Answer from the drawing. Dimensions are ordinates in mm from the lowest x, y and z of the part. A direction names the side the tool comes from. Coordinates: 2 decimals unless noted, no trailing zeros. Order: outer loops, then holes, each group sorted by start corner. A loop starts at its lowest first (then second) coordinate and runs counter-clockwise, first axis right, second up. Notation, with made-up numbers: (34.25, 41.25) - (45.25, 41.25) arc R27 ccw to (45.25, 72.25) - close; hole circle Ø9 at (53, 34.5). An arc over 180 degrees is marked (long way). Use a Markdown table: item, result. Add a question column.
Item 1: The part is cut by section A-A, the plane y = 11.5. Give the vertices of the cut face in (x, z) (1 decimal).
Item 2: Flat-ended cylindrical pins translate along their axes: P1, Ø5, axis at x = 44, z = 42, coming from the -Y side; P2, Ø8, axis at y = 14.5, z = 35, coming from the +X side; P3, Ø2, axis at x = 26.5, z = 53, coming from the -Y side (1 decimal). Find the tip coordinate at first contact, or state that the pin passes through.
Item 3: For the marked faces 4 and 5, determine the directions among +Z, -Z, +X, -X, +Y, -Y from which every point of the face is accessible in a straight line to the end or side of a thin tool.
Item 4: The part is cut by section D-D, the plane y = 15.75. Give the vertices of the cut face in (x, z) (1 decimal).
Item 5: Find the intervals of material crossed by line 1 along Z through (x, y) = (55.5, 25.25); line 2 along Z through (x, y) = (9, 9) (1 decimal); line 3 along X through (y, z) = (23.75, 32.5) (1 decimal), in increasing order.
Item 6: The mould has two halves that part along X. Classify the marked faces 1, 2 and 3: released by +X, released by -X, zero draft, split by the parting line, or undercut.
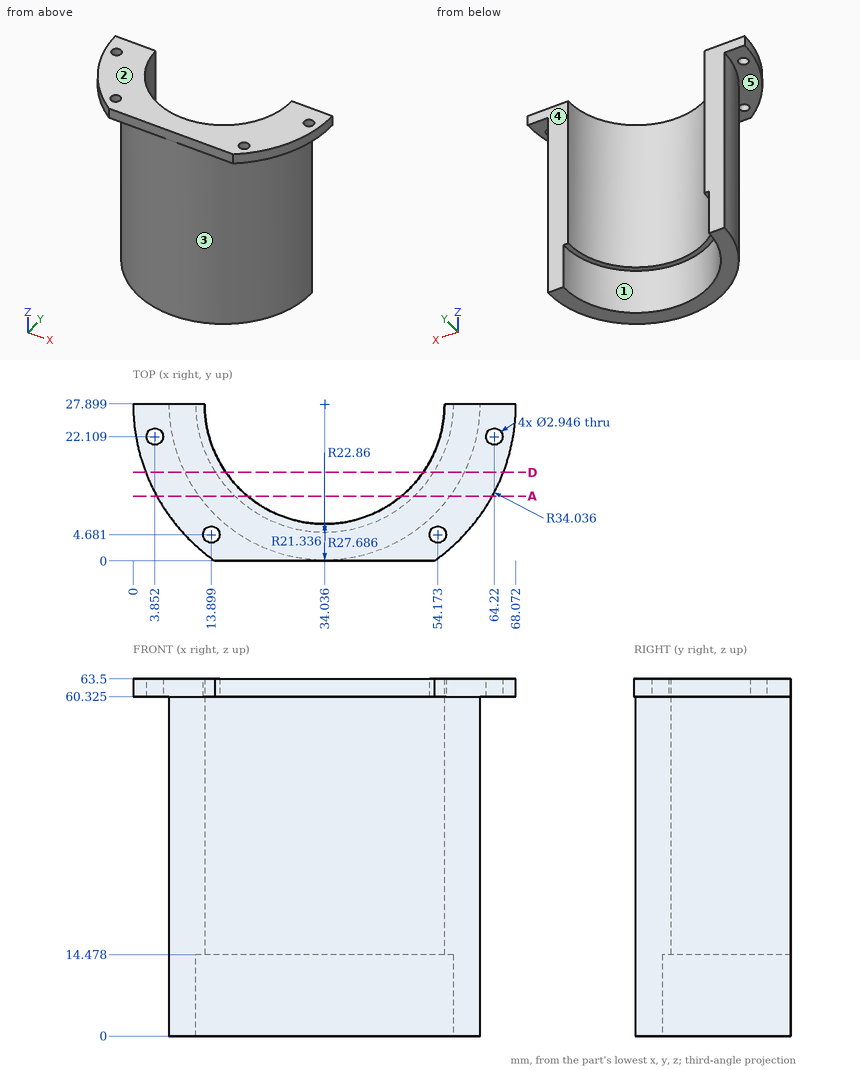
Solution:
| question | item | result |
|---|---|---|
| 1 | outline | (4.2, 60.3) - (11.7, 60.3) - (11.7, 0) - (18.1, 0) - (18.1, 14.5) - (20.4, 14.5) - (20.4, 63.5) - (4.2, 63.5) - close; (47.7, 14.5) - (50, 14.5) - (50, 0) - (56.3, 0) - (56.3, 60.3) - (63.9, 60.3) - (63.9, 63.5) - (47.7, 63.5) - close |
| 2 | P1 | stops at y = 1.24 |
| 2 | P2 | stops at x = 60.08 |
| 2 | P3 | stops at y = 1 |
| 3 | face 4 | +Z, -Z, +X, -X, +Y |
| 3 | face 5 | -Z, -Y |
| 4 | outline | (2.2, 60.3) - (9.2, 60.3) - (9.2, 0) - (14.7, 0) - (14.7, 14.5) - (16.5, 14.5) - (16.5, 63.5) - (2.2, 63.5) - close; (51.6, 14.5) - (53.4, 14.5) - (53.4, 0) - (58.9, 0) - (58.9, 60.3) - (65.8, 60.3) - (65.8, 63.5) - (51.6, 63.5) - close |
| 5 | line 1 | z = 14.48 to 63.5 |
| 5 | line 2 | z = 60.3 to 63.5 |
| 5 | line 3 | x = 6.7 to 13.1, 55 to 61.4 |
| 6 | face 1 | undercut |
| 6 | face 2 | zero draft |
| 6 | face 3 | split by the parting line |
